from build123d import *

# Parameters (mm, degrees)
SKETCH_1_W          = 105
SKETCH_1_H          = 50
EXTRUDE_1_DEPTH     = 2
FILLET_1_R          = 11
SKETCH_3_R          = 2.15
CUT_EXTRUDE_1_DEPTH = 1
CUT_EXTRUDE_2_REACH = 60.157
SKETCH_4_R          = 1.15
CUT_EXTRUDE_3_REACH = 60.183
SKETCH_5_W          = 30.5
SKETCH_5_H          = 29.7


with BuildPart() as part:
    # 草图1 → 凸台-拉伸1 (new body)
    with BuildSketch(Plane.XY):
        Rectangle(SKETCH_1_W, SKETCH_1_H)
    extrude(amount=EXTRUDE_1_DEPTH)

    # 圆角1
    fillet_1_edges = [part.edges().sort_by_distance(p)[0] for p in [
        (52.5, -25, 1),
        (-52.5, -25, 1),
        (-52.5, 25, 1),
        (52.5, 25, 1),
    ]]
    fillet(fillet_1_edges, radius=FILLET_1_R)

    # 草图3 → 切除-拉伸1 (cut)
    with BuildSketch(Plane(origin=(0, 0, 0), x_dir=(-1, 0, 0), z_dir=(0, 0, -1))):
        with Locations((47.88083152, -20)):
            Circle(SKETCH_3_R)
        with Locations((47.88083152, 20)):
            Circle(SKETCH_3_R)
        with Locations((-47.88083152, 20)):
            Circle(SKETCH_3_R)
        with Locations((-47.88083152, -20)):
            Circle(SKETCH_3_R)
    extrude(amount=-CUT_EXTRUDE_1_DEPTH, mode=Mode.SUBTRACT)

    # 草图4 → 切除-拉伸2 (cut, up to next)
    with BuildSketch(Plane(origin=(0, 0, 1), x_dir=(-1, 0, 0), z_dir=(0, 0, -1)), mode=Mode.PRIVATE) as cut_extrude_2_sk1:
        with Locations((47.88083152, -20)):
            Circle(SKETCH_4_R)
    cut_extrude_2_tool1 = extrude(cut_extrude_2_sk1.sketch, amount=-CUT_EXTRUDE_2_REACH, mode=Mode.PRIVATE) & part.part
    # 草图4 → 切除-拉伸2 (cut, up to next)
    with BuildSketch(Plane(origin=(0, 0, 1), x_dir=(-1, 0, 0), z_dir=(0, 0, -1)), mode=Mode.PRIVATE) as cut_extrude_2_sk2:
        with Locations((-47.88083152, -20)):
            Circle(SKETCH_4_R)
    cut_extrude_2_tool2 = extrude(cut_extrude_2_sk2.sketch, amount=-CUT_EXTRUDE_2_REACH, mode=Mode.PRIVATE) & part.part
    # 草图4 → 切除-拉伸2 (cut, up to next)
    with BuildSketch(Plane(origin=(0, 0, 1), x_dir=(-1, 0, 0), z_dir=(0, 0, -1)), mode=Mode.PRIVATE) as cut_extrude_2_sk3:
        with Locations((47.88083152, 20)):
            Circle(SKETCH_4_R)
    cut_extrude_2_tool3 = extrude(cut_extrude_2_sk3.sketch, amount=-CUT_EXTRUDE_2_REACH, mode=Mode.PRIVATE) & part.part
    # 草图4 → 切除-拉伸2 (cut, up to next)
    with BuildSketch(Plane(origin=(0, 0, 1), x_dir=(-1, 0, 0), z_dir=(0, 0, -1)), mode=Mode.PRIVATE) as cut_extrude_2_sk4:
        with Locations((-47.88083152, 20)):
            Circle(SKETCH_4_R)
    cut_extrude_2_tool4 = extrude(cut_extrude_2_sk4.sketch, amount=-CUT_EXTRUDE_2_REACH, mode=Mode.PRIVATE) & part.part
    add(cut_extrude_2_tool1.solids().sort_by_distance((-47.880832, -20, 1))[0], mode=Mode.SUBTRACT)
    add(cut_extrude_2_tool2.solids().sort_by_distance((47.880832, -20, 1))[0], mode=Mode.SUBTRACT)
    add(cut_extrude_2_tool3.solids().sort_by_distance((-47.880832, 20, 1))[0], mode=Mode.SUBTRACT)
    add(cut_extrude_2_tool4.solids().sort_by_distance((47.880832, 20, 1))[0], mode=Mode.SUBTRACT)

    # 草图5 → 切除-拉伸3 (cut, up to next)
    with BuildSketch(Plane(origin=(0, 0, 0), x_dir=(-1, 0, 0), z_dir=(0, 0, -1)), mode=Mode.PRIVATE) as cut_extrude_3_sk1:
        with Locations((2.25, -7.15)):
            Rectangle(SKETCH_5_W, SKETCH_5_H)
    cut_extrude_3_tool1 = extrude(cut_extrude_3_sk1.sketch, amount=-CUT_EXTRUDE_3_REACH, mode=Mode.PRIVATE) & part.part
    add(cut_extrude_3_tool1.solids().sort_by_distance((-2.25, -7.15, 0))[0], mode=Mode.SUBTRACT)


solid = part.part
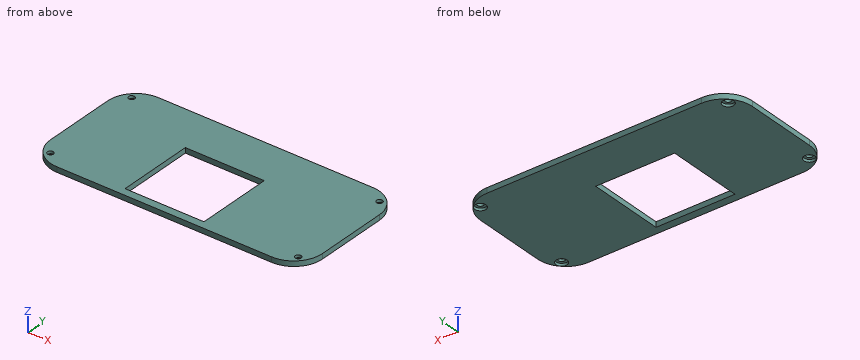
Input: part model. Units: mm. Frame: model coordinates. Round coordinates to 2 decimals unless told otherwise and drop trailing zeros. Loops run counter-clockwise (first coordinate to the right, second up) from the corner with the lowest first, then second, coordinate; pieces in that order, holes last. Notation, with made-up numbers: (89, -37.75) -> (143, -37.75) arc R26 ccw to (143, -9.75) -> close; hole circle Ø2 at (-35.5, 38). An arc over 180 degrees is marked (long way). Answer as a JSON object with one key per item and string values. Group by question number.
1) Section query D-D on y = -15.5. Output: boundary loops of the cut face in (x, z).
2) Section query B-B on z = 1.7. Output: boundary loops of the cut face in (x, y), plus the area to 3 significant figures.
3) Ray query, L1, parallel to Y at x = 9.5, z = 1.4; L2, parallel to X at y = -1.5, z = 0.1; L3, parallel to X at y = -21.5, z = 1.85. Return the intervals inside material, ascending.
4) Section query A-A on x = 11. Output: boundary loops of the cut face in (y, z).
5) Pin query (flat end, axial travel): pin 1 (2.5 mm diameter, centred on x = -47.88, y = 20, fed in from -Z). Return the tip coordinate at first contact, or that it passes through.
6) Section query C-C on y = 20. Output: boundary loops of the cut face in (x, z), plus the area to 3 significant figures.
Reply:
{
 "1": {"outline": "(-52.4, 0) -> (-17.5, 0) -> (-17.5, 2) -> (-52.4, 2) -> close; (13, 0) -> (52.4, 0) -> (52.4, 2) -> (13, 2) -> close"},
 "2": {"outline": "(-52.5, -14) arc R11 ccw to (-41.5, -25) -> (41.5, -25) arc R11 ccw to (52.5, -14) -> (52.5, 14) arc R11 ccw to (41.5, 25) -> (-41.5, 25) arc R11 ccw to (-52.5, 14) -> close; hole circle Ø2.3 at (-47.88, -20); hole circle Ø2.3 at (-47.88, 20); hole (-17.5, -22) -> (13, -22) -> (13, 7.7) -> (-17.5, 7.7) -> close; hole circle Ø2.3 at (47.88, -20); hole circle Ø2.3 at (47.88, 20)", "area": "4,220 mm2"},
 "3": {"L1": "y = -25 to -22, 7.7 to 25", "L2": "x = -52.5 to -17.5, 13 to 52.5", "L3": "x = -49.55 to -17.5, 13 to 49.55"},
 "4": {"outline": "(-25, 0) -> (-22, 0) -> (-22, 2) -> (-25, 2) -> close; (7.7, 0) -> (25, 0) -> (25, 2) -> (7.7, 2) -> close"},
 "5": {"pin 1": "stops at z = 1"},
 "6": {"outline": "(-50.72, 0) -> (-50.03, 0) -> (-50.03, 1) -> (-49.03, 1) -> (-49.03, 2) -> (-50.72, 2) -> close; (-46.73, 1) -> (-45.73, 1) -> (-45.73, 0) -> (45.73, 0) -> (45.73, 1) -> (46.73, 1) -> (46.73, 2) -> (-46.73, 2) -> close; (49.03, 1) -> (50.03, 1) -> (50.03, 0) -> (50.72, 0) -> (50.72, 2) -> (49.03, 2) -> close", "area": "190 mm2"}
}
